Geometry: see drawing. Coordinates: mm, zero at the bounding-box minimum. Coordinates: 2 decimals unless noted, no trailing zeros. Order: outer loops, then holes, each group sorted by start corner. A loop starts at its lowest first (then second) coordinate and runs counter-clockwise, first axis right, second up.
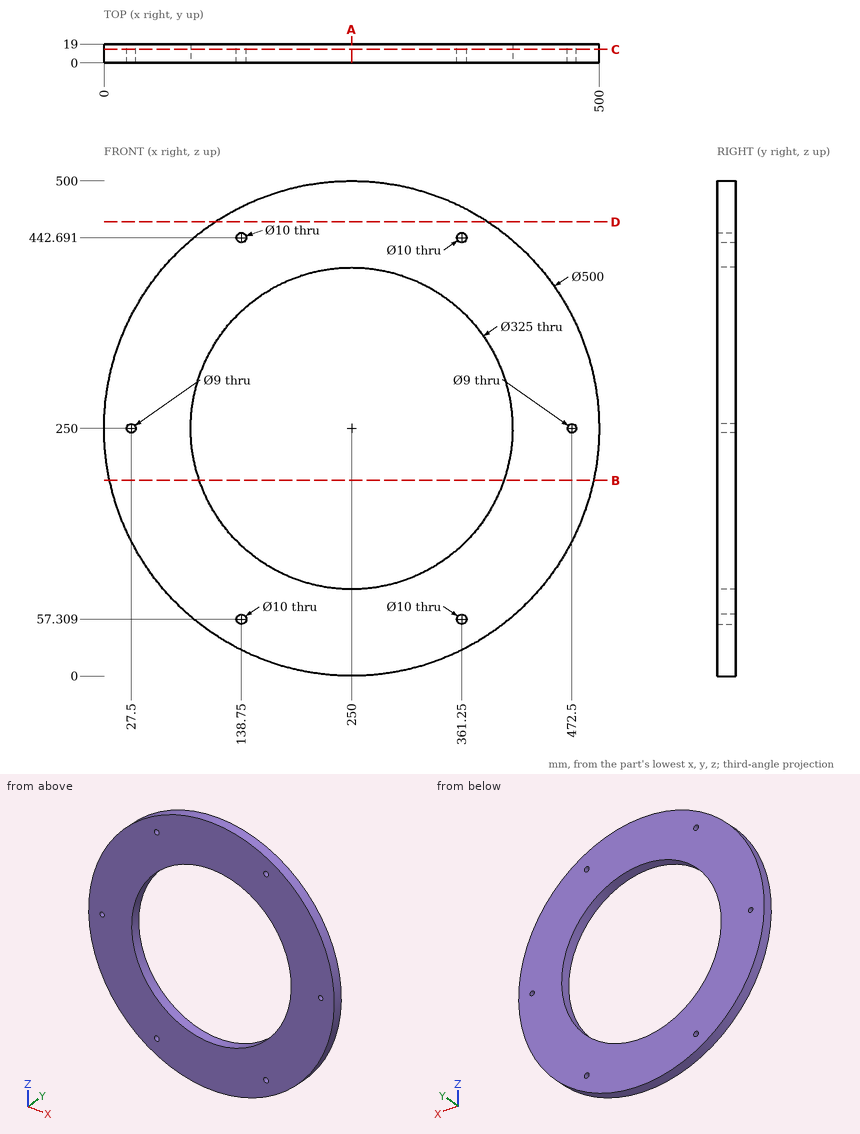
Item 1: Cut plane A-A on x = 250. Return loops of the section in (y, z), then the cut area to 4 significant figures.
Response values:
outline: (0, 0) - (19, 0) - (19, 87.5) - (0, 87.5) - close; (0, 412.5) - (19, 412.5) - (19, 500) - (0, 500) - close
area: 3,325 mm2
Item 2: Cut plane D-D on z = 458.5. Return loops of the section in (x, y).
Response values:
outline: (112.06, 0) - (387.94, 0) - (387.94, 19) - (112.06, 19) - close
Item 3: Cut plane C-C on y = 13.5. Return loops of the section in (x, z), then the cut area to 3 significant figures.
Response values:
outline: circle Ø500 at (250, 250); hole circle Ø9 at (27.5, 250); hole circle Ø325 at (250, 250); hole circle Ø10 at (138.75, 57.31); hole circle Ø10 at (138.75, 442.69); hole circle Ø10 at (361.25, 57.31); hole circle Ø10 at (361.25, 442.69); hole circle Ø9 at (472.5, 250)
area: 113,000 mm2
Item 4: Ray query, probe 1 along X at (y, z) = (11, 250); probe 2 along Z at (x, y) = (361.25, 12.25) (1 decimal); probe 3 along Z at (x, y) = (375.5, 3) (1 decimal). Return the intervals inside material, ascending.
Response values:
probe 1: x = 0 to 23, 32 to 87.5, 412.5 to 468, 477 to 500
probe 2: z = 26.1 to 52.3, 62.3 to 131.6, 368.4 to 437.7, 447.7 to 473.9
probe 3: z = 33.8 to 146.8, 353.2 to 466.2
Item 5: Pin query (flat end, axial travel): pin 1 Ø8 at (y, z) = (10, 220) entering from +X; pin 2 Ø1.5 at (x, y) = (171.5, 11.5) entering from +Z; pin 3 Ø3 at (x, y) = (187.5, 10.5) entering from -Z. Return the tip coordinate at first contact, or that it passes through.
Response values:
pin 1: stops at x = 498.64
pin 2: stops at z = 487.6
pin 3: stops at z = 7.56
Item 6: Cut plane B-B on z = 197.5. Return loops of the section in (x, y) (1 decimal), then the cut area to 3 significant figures.
Response values:
outline: (5.6, 0) - (96.2, 0) - (96.2, 19) - (5.6, 19) - close; (403.8, 0) - (494.4, 0) - (494.4, 19) - (403.8, 19) - close
area: 3,440 mm2
